```python
from build123d import *

# Parameters (mm, degrees)
SKETCH5_R                    = 16.51
CUT_EXTRUDE2_DEPTH           = 19.304
CUT_EXTRUDE2_DEPTH_BACK      = 110.744
SKETCH2_R                    = 7.62
CUT_EXTRUDE3_DEPTH           = 1.905
CUT_EXTRUDE3_TAPER           = 45
CUT_EXTRUDE3_OTHER_WAY_DEPTH = 9.398
SKETCH9_R                    = 7.62
CUT_EXTRUDE5_DEPTH           = 1.905
CUT_EXTRUDE5_TAPER           = 45
CUT_EXTRUDE5_OTHER_WAY_DEPTH = 127
SKETCH10_R                   = 5.715
CUT_EXTRUDE6_DEPTH           = 1.905
CUT_EXTRUDE6_DEPTH_BACK      = 48.641


with BuildPart() as part:
    # Sketch1 → Revolve1 (revolve)
    with BuildSketch(Plane(origin=(0, 0, 0), x_dir=(1, 0, 0), z_dir=(0, 1, 0))):
        with BuildLine():
            Line((0, 0), (4.988818102, 2.880295474))
            ThreePointArc((4.988818102, 2.880295474), (6.258818102, 5.08), (4.988818102, 7.279704526))
            Line((4.988818102, 7.279704526), (0, 10.16))
            Line((0, 10.16), (0, 11.555300166))
            Line((0, 11.555300166), (41.91, 11.555300166))
            Line((41.91, 11.555300166), (41.91, -1.144699834))
            Line((41.91, -1.144699834), (0, -1.144699834))
            Line((0, -1.144699834), (0, 0))
        make_face()
    revolve(axis=Axis((41.91, 0, -11.555300166), (0, 0, 1)))

    # Sketch5 → Cut-Extrude2 (cut, two sides)
    with BuildSketch(Plane.XY.offset(1.144699834)) as cut_extrude2_sk:
        with Locations((41.91, 0)):
            Circle(SKETCH5_R)
    extrude(amount=CUT_EXTRUDE2_DEPTH, mode=Mode.SUBTRACT)
    extrude(cut_extrude2_sk.sketch, amount=-CUT_EXTRUDE2_DEPTH_BACK, mode=Mode.SUBTRACT)

    # Sketch2 → Cut-Extrude3 (cut)
    with BuildSketch(Plane.XY):
        with Locations((67.31, 0)):
            Circle(SKETCH2_R)
        with Locations((61.367528855, -16.326805286)):
            Circle(SKETCH2_R)
        with Locations((61.367528855, 16.326805286)):
            Circle(SKETCH2_R)
        with Locations((46.320663713, 25.014116927)):
            Circle(SKETCH2_R)
        with Locations((29.21, 21.997045256)):
            Circle(SKETCH2_R)
        with Locations((18.041807432, 8.68731164)):
            Circle(SKETCH2_R)
        with Locations((18.041807432, -8.68731164)):
            Circle(SKETCH2_R)
        with Locations((29.21, -21.997045256)):
            Circle(SKETCH2_R)
        with Locations((46.320663713, -25.014116927)):
            Circle(SKETCH2_R)
    extrude(amount=-CUT_EXTRUDE3_DEPTH, taper=CUT_EXTRUDE3_TAPER, mode=Mode.SUBTRACT)

    # Sketch2 → Cut-Extrude3 other way (cut)
    with BuildSketch(Plane.XY):
        with Locations((67.31, 0)):
            Circle(SKETCH2_R)
        with Locations((61.367528855, -16.326805286)):
            Circle(SKETCH2_R)
        with Locations((61.367528855, 16.326805286)):
            Circle(SKETCH2_R)
        with Locations((46.320663713, 25.014116927)):
            Circle(SKETCH2_R)
        with Locations((29.21, 21.997045256)):
            Circle(SKETCH2_R)
        with Locations((18.041807432, 8.68731164)):
            Circle(SKETCH2_R)
        with Locations((18.041807432, -8.68731164)):
            Circle(SKETCH2_R)
        with Locations((29.21, -21.997045256)):
            Circle(SKETCH2_R)
        with Locations((46.320663713, -25.014116927)):
            Circle(SKETCH2_R)
    extrude(amount=CUT_EXTRUDE3_OTHER_WAY_DEPTH, mode=Mode.SUBTRACT)

    # Sketch9 → Cut-Extrude5 (cut)
    with BuildSketch(Plane(origin=(0, 0, -11.555300166), x_dir=(-1, 0, 0), z_dir=(0, 0, -1))):
        with Locations((-67.31, 0)):
            Circle(SKETCH9_R)
        with Locations((-61.367528855, 16.326805286)):
            Circle(SKETCH9_R)
        with Locations((-46.320663713, 25.014116927)):
            Circle(SKETCH9_R)
        with Locations((-29.21, 21.997045256)):
            Circle(SKETCH9_R)
        with Locations((-18.041807432, 8.68731164)):
            Circle(SKETCH9_R)
        with Locations((-18.041807432, -8.68731164)):
            Circle(SKETCH9_R)
        with Locations((-29.21, -21.997045256)):
            Circle(SKETCH9_R)
        with Locations((-46.320663713, -25.014116927)):
            Circle(SKETCH9_R)
        with Locations((-61.367528855, -16.326805286)):
            Circle(SKETCH9_R)
    extrude(amount=-CUT_EXTRUDE5_DEPTH, taper=CUT_EXTRUDE5_TAPER, mode=Mode.SUBTRACT)

    # Sketch9 → Cut-Extrude5 other way (cut)
    with BuildSketch(Plane(origin=(0, 0, -11.555300166), x_dir=(-1, 0, 0), z_dir=(0, 0, -1))):
        with Locations((-67.31, 0)):
            Circle(SKETCH9_R)
        with Locations((-61.367528855, 16.326805286)):
            Circle(SKETCH9_R)
        with Locations((-46.320663713, 25.014116927)):
            Circle(SKETCH9_R)
        with Locations((-29.21, 21.997045256)):
            Circle(SKETCH9_R)
        with Locations((-18.041807432, 8.68731164)):
            Circle(SKETCH9_R)
        with Locations((-18.041807432, -8.68731164)):
            Circle(SKETCH9_R)
        with Locations((-29.21, -21.997045256)):
            Circle(SKETCH9_R)
        with Locations((-46.320663713, -25.014116927)):
            Circle(SKETCH9_R)
        with Locations((-61.367528855, -16.326805286)):
            Circle(SKETCH9_R)
    extrude(amount=CUT_EXTRUDE5_OTHER_WAY_DEPTH, mode=Mode.SUBTRACT)

    # Sketch10 → Cut-Extrude6 (cut, two sides)
    with BuildSketch(Plane.XY.offset(1.144699834)) as cut_extrude6_sk:
        with Locations((29.21, 21.997045256)):
            Circle(SKETCH10_R)
        with Locations((46.320663713, 25.014116927)):
            Circle(SKETCH10_R)
        with Locations((61.367528855, 16.326805286)):
            Circle(SKETCH10_R)
        with Locations((67.31, 0)):
            Circle(SKETCH10_R)
        with Locations((61.367528855, -16.326805286)):
            Circle(SKETCH10_R)
        with Locations((46.320663713, -25.014116927)):
            Circle(SKETCH10_R)
        with Locations((29.21, -21.997045256)):
            Circle(SKETCH10_R)
        with Locations((18.041807432, -8.68731164)):
            Circle(SKETCH10_R)
        with Locations((18.041807432, 8.68731164)):
            Circle(SKETCH10_R)
    extrude(amount=CUT_EXTRUDE6_DEPTH, mode=Mode.SUBTRACT)
    extrude(cut_extrude6_sk.sketch, amount=-CUT_EXTRUDE6_DEPTH_BACK, mode=Mode.SUBTRACT)


solid = part.part
```
Here's how the part is built. I have some questions about the finished solid (model axes, mm). A direction names the side the tool comes from. Round coordinates to 2 decimals unless told otherwise and drop trailing zeros. Answer as CSV lines item,"result".
Item 1: Which directions (+Z, -Z, +X, -X, +Y, -Y) give clear straight access to the entire face, cutting with the end or side of a thin tool? Please do faces 1 (the cylindrical face through (32.282, -17.178, -5.723)), 2 (the conical face through (6.46, -11.16, -2.74)), 3 (the cylindrical face through (74.35, -2.92, 0.56)).
From the geometry:
face 1,"+Z, -Z"
face 2,"none"
face 3,"+Z"
Item 2: Please list where these lines run through material, in increasing order: L1, parallel to Y at x = 61.5, z = -3; L2, parallel to Y at x = 29.21, z = 0.8; L3, parallel to Y at x = 67.31, z = 0.45. Write a range as [from, to].
From the geometry:
L1,"[-31.07, -22.04], [-10.61, 10.61], [22.04, 31.07]"
L2,"[-39.94, -29.62], [-14.38, -10.55], [10.55, 14.38], [29.62, 39.94]"
L3,"[-33.34, -21.1], [-11.56, -7.62], [7.62, 11.56], [21.1, 33.34]"
Item 3: Imagine slicing it at A-A on y = 0. Give the number of separate pieces and of enclosed holes in the cut face, and give its area (3 significant figures).
From the geometry:
separate pieces,"3"
enclosed holes,"0"
area,"408 mm2"
Item 4: We'd pull the mould along Y, two halves only. Please class faces 4 (the flat face through (42, 18, -11.555)), 5 (the cylindrical face through (83.78, -1.84, 0.56)), 6 (the cylindrical face through (11.99, -13.32, 0.56)): +Y half, -Y half, draft (parallel to the pull), parting line (faces both ways), or undercut.
From the geometry:
face 4,"draft"
face 5,"parting line"
face 6,"undercut"
Item 5: For pin 1 (9 mm diameter, centred on x = 29.21, y = -22, fed in from +Z); pin 2 (3 mm diameter, centred on x = 17, z = -9.5, fed in from +Y); pin 3 (13.5 mm diameter, centred on x = 46.32, y = 25.01, fed in from -Z); pin 4 (2 mm diameter, centred on y = -8, z = -6.5, fed in from -X), each with a flat end and sliding along its axis, tell me the tip position at first contact or that it passes through.
From the geometry:
pin 1,"through"
pin 2,"y = 34.66"
pin 3,"z = -10.69"
pin 4,"x = 5.46"
